Input: part model. Units: mm. Frame: model coordinates. A direction names the side the tool comes from. Coordinates: 2 decimals unless noted, no trailing zeros. Write each loop counter-clockwise with the first axis right and the second up, starting at its lowest first coordinate (ties: lowest second). Pieces come first, ordered by that corner, then holes. Notation, with made-up numbers: (45, -4.75) - (101, -4.75) arc R14 cw to (101, 15.25) - close; hole circle Ø11 at (-26, -34.5). An arc over 180 degrees is marked (long way). Use a Markdown table: item, result. Add a question column.
Q1. Mould query, pull axis Y, two halves, no side actions, for faces 1 (the face through (0, 60, 26)), 2 (the face through (0, 30, 40.026)), 3 (the face through (0, 30, 34.526)). Classes: released by +Y, released by -Y, zero draft, split by the parting line, or undercut.
Q2. Section query C-C (y = 21.5). Return the cut outline in (x, z) (1 decimal).
Q3. Pin query (flat end, axial travel): P1, Ø0.6, axis at y = 38, z = 8.5, coming from the -X side (3 decimals); P2, Ø1.8, axis at y = 10, z = 25.03, coming from the +X side; P3, Ø1.7, axis at x = -6, y = 27, coming from the -Z side; P4, Ø0.7, axis at x = 3.5, y = 40, coming from the -Z side. Return the tip coordinate at first contact, or that it passes through.
Q4. Material intervals for probe 1 along Z at (x, y) = (2.5, 30); probe 2 along Z at (x, y) = (5.75, 23); probe 3 along Y at (x, z) = (5, 20.5), sorted ascending. Write a range as from..to.
Q5. Section query A-A (y = 10). Return the cut outline in (x, z) (1 decimal), then the cut area to 3 significant figures.
Q6. Set-up query: faces 4 (the face through (4, 30, 7.96)), 5 (the face through (5.242, 30, 7)), 6 (the face through (-0.14, 43.072, 15.977)). Return all of +Z, -Z, +X, -X, +Y, -Y with unobstructed straight access to the full face (end or side cutting, diameter ignored); none if empty.
Q7. Section query B-B (x = 8.5). Return the cut outline in (y, z), then the cut area to 3 significant figures.
Autodesk Fusion 360 part; units mm, degrees
sketch "Sketch1" plane through (0, 0, 0) normal (0, 1, 0) x (1, 0, 0)
  line L0 (2.8825, -8.6547) -> (4.3945, -10.1667)
  line L1 (3.9, -0.21) -> (3.9, -2.8393)
  line L2 (-8.2, 5.5) -> (-8.2, 3.125)
  line L3 (-2.925, -8.676) -> (-4.4001, -10.1511)
  arc A0 (9.4998, -10.0253) -> (10.0042, -9.4999) centre (9.4925, -9.5135) ccw
  line L4 (0, -4.0611) -> (-0.1019, -4.163)
  line L5 (5.5, 8.2) -> (3.125, 8.2)
  line L6 (-6.5607, -5.5) -> (-8.2, -5.5)
  line L7 (5.2425, -6.658) -> (5.2425, -7.96)
  line L8 (-8.2, -5.5) -> (-8.2, -3.1249)
  line L9 (0, -4.0611) -> (0.1019, -4.163)
  line L10 (-2.7368, -4.163) -> (-5.2537, -6.6799)
  line L11 (-3.125, 8.545) -> (-4.58, 10)
  line L12 (6.5607, 5.5) -> (8.2, 5.5)
  line L13 (-3.125, 8.2) -> (-3.125, 8.545)
  arc A1 (-9.5, 10) -> (-10, 9.5) centre (-9.5, 9.5) ccw
  line L14 (8.2, 3.125) -> (8.545, 3.125)
  line L15 (-3.9, 0.21) -> (-3.9, 2.8393)
  line L16 (-10, 9.5) -> (-10, 4.58)
  line L17 (0.1019, -4.163) -> (2.7475, -4.163)
  line L18 (-3.125, -8.14) -> (-3.125, -8.5931)
  line L19 (-6.5607, 5.5) -> (-8.2, 5.5)
  line L20 (-5.2537, -7.94) -> (-2.925, -7.94)
  line L21 (3.69, 0) -> (3.9, -0.21)
  line L22 (-10.0013, -4.5807) -> (-10.0013, -9.5)
  line L23 (-0.1019, -4.163) -> (-2.7368, -4.163)
  line L24 (-3.69, 0) -> (-3.9, -0.21)
  line L25 (3.9, -2.8393) -> (6.5607, -5.5)
  line L26 (-5.4537, -6.5971) -> (-5.4537, -8.14)
  arc A2 (10, 9.5) -> (9.5, 10) centre (9.5, 9.5) ccw
  line L27 (-3.9, 2.8393) -> (-6.5607, 5.5)
  line L28 (8.545, 3.125) -> (10, 4.58)
  line L29 (10.0042, -4.5823) -> (10.0042, -9.4999)
  line L30 (-5.4537, -8.14) -> (-3.125, -8.14)
  line L31 (-10, -10.0258) -> (-10, -15)
  line L32 (-3.125, -8.5931) -> (-4.5415, -10.0097)
  line L33 (-3.9, -2.8393) -> (-6.5607, -5.5)
  line L34 (3.0825, -8.5719) -> (4.5359, -10.0253)
  line L35 (5.4425, -8.16) -> (3.0825, -8.16)
  line L36 (-2.925, -7.94) -> (-2.925, -8.676)
  line L37 (3.125, 8.2) -> (3.125, 8.545)
  line L38 (8.2, -3.1245) -> (8.5464, -3.1245)
  line L39 (8.2, -5.5) -> (8.2, -3.1245)
  line L40 (0, -3.7782) -> (0.1847, -3.963)
  line L41 (0, -3.7782) -> (-0.1847, -3.963)
  line L42 (0.1847, -3.963) -> (2.8304, -3.963)
  line L43 (-9.5, -10.0097) -> (-4.5415, -10.0097)
  line L44 (4.5359, -10.0253) -> (9.4998, -10.0253)
  line L45 (6.5607, -5.5) -> (8.2, -5.5)
  line L46 (-2.8196, -3.963) -> (-5.4537, -6.5971)
  line L47 (-8.2, -3.1249) -> (-8.5454, -3.1249)
  line L48 (8.5464, -3.1245) -> (10.0042, -4.5823)
  arc A3 (-10.0013, -9.5) -> (-9.5, -10.0097) centre (-9.4969, -9.5053) ccw
  line L49 (10, -15) -> (10, -10.0258)
  line L50 (-5.2537, -6.6799) -> (-5.2537, -7.94)
  line L51 (5.2425, -7.96) -> (2.8825, -7.96)
  line L52 (3.0825, -8.16) -> (3.0825, -8.5719)
  line L53 (5.4425, -6.5751) -> (5.4425, -8.16)
  line L54 (3.9, 0.21) -> (3.9, 2.8393)
  line L55 (-3.9, -0.21) -> (-3.9, -2.8393)
  line L56 (3.9, 2.8393) -> (6.5607, 5.5)
  line L57 (-5.5, 6.5607) -> (-5.5, 8.2)
  line L58 (2.8825, -7.96) -> (2.8825, -8.6547)
  line L59 (-8.5454, -3.1249) -> (-10.0013, -4.5807)
  line L60 (0, 3.69) -> (-0.21, 3.9)
  line L61 (2.8304, -3.963) -> (5.4425, -6.5751)
  line L62 (2.7475, -4.163) -> (5.2425, -6.658)
  line L63 (-8.545, 3.125) -> (-10, 4.58)
  line L64 (-0.1847, -3.963) -> (-2.8196, -3.963)
  line L65 (5.5, 6.5607) -> (5.5, 8.2)
  line L66 (-0.21, 3.9) -> (-2.8393, 3.9)
  line L67 (3.69, 0) -> (3.9, 0.21)
  line L68 (-5.5, 8.2) -> (-3.125, 8.2)
  line L69 (-8.2, 3.125) -> (-8.545, 3.125)
  line L70 (-2.8393, 3.9) -> (-5.5, 6.5607)
  line L71 (2.8393, 3.9) -> (5.5, 6.5607)
  line L72 (10, 9.5) -> (10, 4.58)
  line L73 (8.2, 5.5) -> (8.2, 3.125)
  line L74 (-3.69, 0) -> (-3.9, 0.21)
  line L75 (0.21, 3.9) -> (2.8393, 3.9)
  line L76 (4.58, 10) -> (9.5, 10)
  circle A4 centre (0, 0) radius 2.5
  line L77 (3.125, 8.545) -> (4.58, 10)
  line L78 (-9.5, 10) -> (-4.58, 10)
  line L79 (0, 3.69) -> (0.21, 3.9)
  line L80 (-10, -15) -> (10, -15)
  line L81 (0.1019, -4.163) -> (-0.1019, -4.163)
  line L82 (4.2531, -10.0253) -> (4.5359, -10.0253)
  line L83 (10, -10.0258) -> (4.2536, -10.0258)
  line L84 (-4.2748, -10.0258) -> (-10, -10.0258)
  line L85 (2.8825, -8.6547) -> (2.8825, -10.0258)
  line L86 (2.8825, -10.0258) -> (4.2536, -10.0258)
  line L87 (-2.925, -8.676) -> (-2.925, -10.0353)
  line L88 (-2.925, -10.0353) -> (-4.2748, -10.0258)
  point P0 (0, -10)
  dimension "d1" = 0.2
  dimension "d2" = 5
extrude "Extrude1" add sketch "Sketch1" along normal blind 60 contours L7 L10 L17 L20 L23 L31 L36 L44 L49 L50 L51 L58 L62 L80 L81 L82 L83 L84 L85 L86 L87 L88
sketch "Sketch2" plane through (10, 0, 0) normal (1, 0, 0) x (0, 1, 0)
  line L0 (0, 15) -> (0, 10.0258)
  line L1 (0, 10.0258) -> (60, 10.0258)
  line L2 (60, 10.0258) -> (60, 15)
  line L3 (60, 15) -> (0, 15)
  line L4 (0, 10.0258) -> (60, 10.0258)
  line L5 (60, 10.0258) -> (60, 40.0258)
  line L6 (60, 40.0258) -> (0, 40.0258)
  line L7 (0, 40.0258) -> (0, 10.0258)
  line L8 (60, 40.0258) -> (0, 10.0258) construction
  line L9 (0, 40.0258) -> (60, 10.0258) construction
  line L10 (43.5, 34.5258) -> (16.5, 34.5258)
  line L11 (16.5, 34.5258) -> (16.5, 15.5258)
  line L12 (16.5, 15.5258) -> (43.5, 15.5258)
  line L13 (43.5, 15.5258) -> (43.5, 34.5258)
  line L14 (43.5, 34.5258) -> (16.5, 15.5258) construction
  line L15 (16.5, 34.5258) -> (43.5, 15.5258) construction
  line L16 (16.5, 25.0258) -> (10, 25.0258)
  line L17 (43.5, 25.0258) -> (50, 25.0258)
  circle A0 centre (10, 25.0258) radius 1
  circle A1 centre (50, 25.0258) radius 1
  point P0 (30, 25.0258)
  dimension "d5" = 30
  dimension "d6" = 60
  dimension "d7" = 27
  dimension "d8" = 19
  dimension "d9" = 6.5
  dimension "d10" = 6.5
  dimension "d11" = 2
  dimension "d12" = 2
extrude "Extrude2" add sketch "Sketch2" against normal blind 20 contours L3 L5 L6 L7
fillet "Fillet1" radius 1.5 4 edges at (0, 43.5, 15.5258) (0, 16.5, 15.5258) (0, 43.5, 34.5258) (0, 16.5, 34.5258)
Values follow:
| question | item | result |
|---|---|---|
| 1 | face 1 | released by +Y |
| 1 | face 2 | zero draft |
| 1 | face 3 | undercut |
| 2 | outline | (-10, 10) - (-4.3, 10) - (-2.9, 10) - (-2.9, 7.9) - (-5.3, 7.9) - (-5.3, 6.7) - (-2.7, 4.2) - (2.7, 4.2) - (5.2, 6.7) - (5.2, 8) - (2.9, 8) - (2.9, 10) - (4.3, 10) - (9.5, 10) - (10, 10) - (10, 15.5) - (-10, 15.5) - close; (-10, 34.5) - (10, 34.5) - (10, 40) - (-10, 40) - close |
| 3 | P1 | x = -2.925 |
| 3 | P2 | through |
| 3 | P3 | z = 6.58 |
| 3 | P4 | z = 4.57 |
| 4 | probe 1 | 4.16..15.53, 34.53..40.03 |
| 4 | probe 2 | 10.03..15.53, 34.53..40.03 |
| 4 | probe 3 | 0..16.5, 43.5..60 |
| 5 | outline | (-10, 10) - (-4.3, 10) - (-2.9, 10) - (-2.9, 7.9) - (-5.3, 7.9) - (-5.3, 6.7) - (-2.7, 4.2) - (2.7, 4.2) - (5.2, 6.7) - (5.2, 8) - (2.9, 8) - (2.9, 10) - (4.3, 10) - (9.5, 10) - (10, 10) - (10, 24) - (-10, 24) - close; (-10, 26) - (10, 26) - (10, 40) - (-10, 40) - close |
| 5 | area | 606 mm2 |
| 6 | face 4 | +X, +Y, -Y |
| 6 | face 5 | -Z, +X, +Y, -Y |
| 6 | face 6 | +X, -X |
| 7 | outline | (0, 10.03) - (60, 10.03) - (60, 40.03) - (0, 40.03) - close; hole circle Ø2 at (10, 25.03); hole (16.5, 17.03) arc R1.5 ccw to (18, 15.53) - (42, 15.53) arc R1.5 ccw to (43.5, 17.03) - (43.5, 33.03) arc R1.5 ccw to (42, 34.53) - (18, 34.53) arc R1.5 ccw to (16.5, 33.03) - close; hole circle Ø2 at (50, 25.03) |
| 7 | area | 1,280 mm2 |
